Geometry: final body of the model. Coordinates: model frame, mm. Face numbers are marked on the shaded views. A direction names the side the tool comes from. Round coordinates to 2 decimals unless told otherwise and drop trailing zeros. Loops run counter-clockwise (first coordinate to the right, second up) from the corner with the lowest first, then second, coordinate; pieces in that order, holes last. Notation, with made-up numbers: (67, 89) -> (125, 89) arc R23 cw to (125, 112) -> close; hole circle Ø6 at (59.5, 40). An arc over 180 degrees is marked (long way). Answer in a Markdown table with one row per item.
```python
from build123d import *

# Parameters (mm, degrees)
BOSS_EXTRUDE1_DEPTH      = 1.5
BOSS_EXTRUDE2_DEPTH      = 6
BOSS_EXTRUDE2_DEPTH_BACK = 3
CUT_EXTRUDE1_DEPTH       = 13.69206445
CUT_EXTRUDE1_DEPTH_BACK  = 13.69206445


with BuildPart() as part:
    # Sketch1 → Boss-Extrude1 (new body)
    with BuildSketch(Plane(origin=(0, 0, 0), x_dir=(1, 0, 0), z_dir=(0, 1, 0))):
        Polygon((-0.635, 10.16), (0.635, 10.16), (1.27, 9.525), (1.27, 8.255), (0.635, 7.62), (1.27, 6.985), (1.27, 5.715), (0.635, 5.08), (1.27, 4.445), (1.27, 3.175), (0.635, 2.54), (1.27, 1.905), (1.27, 0.635), (0.635, 0), (1.27, -0.635), (1.27, -1.905), (0.635, -2.54), (1.27, -3.175), (1.27, -4.445), (0.635, -5.08), (-0.635, -5.08), (-1.27, -4.445), (-1.27, -3.175), (-0.635, -2.54), (-1.27, -1.905), (-1.27, -0.635), (-0.635, 0), (-1.27, 0.635), (-1.27, 1.905), (-0.635, 2.54), (-1.27, 3.175), (-1.27, 4.445), (-0.635, 5.08), (-1.27, 5.715), (-1.27, 6.985), (-0.635, 7.62), (-1.27, 8.255), (-1.27, 9.525), align=None)
    extrude(amount=BOSS_EXTRUDE1_DEPTH)

    # Sketch3 → Boss-Extrude2 (add, two sides: drawn at the far end of the back side and taken through both)
    with BuildSketch(Plane(origin=(0, 1.5, 0), x_dir=(1, 0, 0), z_dir=(0, 1, 0)).offset(-BOSS_EXTRUDE2_DEPTH_BACK)):
        Polygon((0.375, 9.39), (0.5, 9.265), (0.5, 8.515), (0.375, 8.39), (-0.375, 8.39), (-0.5, 8.515), (-0.5, 9.265), (-0.375, 9.39), align=None)
        Polygon((0.375, 6.85), (0.5, 6.725), (0.5, 5.975), (0.375, 5.85), (-0.375, 5.85), (-0.5, 5.975), (-0.5, 6.725), (-0.375, 6.85), align=None)
        Polygon((0.375, 4.31), (0.5, 4.185), (0.5, 3.435), (0.375, 3.31), (-0.375, 3.31), (-0.5, 3.435), (-0.5, 4.185), (-0.375, 4.31), align=None)
        Polygon((0.375, 1.77), (0.5, 1.645), (0.5, 0.895), (0.375, 0.77), (-0.375, 0.77), (-0.5, 0.895), (-0.5, 1.645), (-0.375, 1.77), align=None)
        Polygon((0.375, -0.77), (0.5, -0.895), (0.5, -1.645), (0.375, -1.77), (-0.375, -1.77), (-0.5, -1.645), (-0.5, -0.895), (-0.375, -0.77), align=None)
        Polygon((0.375, -3.31), (0.5, -3.435), (0.5, -4.185), (0.375, -4.31), (-0.375, -4.31), (-0.5, -4.185), (-0.5, -3.435), (-0.375, -3.31), align=None)
    extrude(amount=BOSS_EXTRUDE2_DEPTH + BOSS_EXTRUDE2_DEPTH_BACK)

    # Sketch4 → Cut-Extrude1 (cut, two sides: drawn at the far end of the back side and taken through both)
    with BuildSketch(Plane(origin=(0, 0, 0), x_dir=(1, 0, 0), z_dir=(0, 1, 0)).offset(-CUT_EXTRUDE1_DEPTH_BACK)):
        Polygon((0.635, 2.54), (-0.635, 2.54), (-3.551273802, 2.145414022), (-3.551273802, -5.54901255), (3.518391637, -6.305302341), (3.518391637, 1.323359901), align=None)
    extrude(amount=CUT_EXTRUDE1_DEPTH + CUT_EXTRUDE1_DEPTH_BACK, mode=Mode.SUBTRACT)


solid = part.part
```
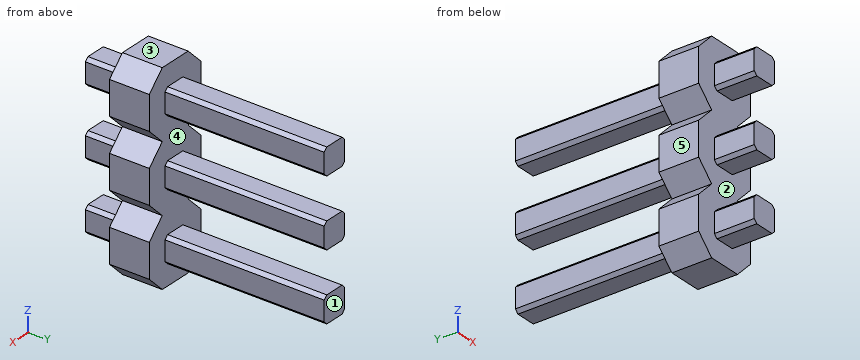
Item 1: Section query D-D, the plane z = -4. Output: boundary loops of the cut face in (x, y), and give its area (3 significant figures).
Ans:
| item | result |
|---|---|
| outline | (-1.27, 0) -> (-0.5, 0) -> (-0.5, -1.5) -> (0.5, -1.5) -> (0.5, 0) -> (1.27, 0) -> (1.27, 1.5) -> (0.5, 1.5) -> (0.5, 7.5) -> (-0.5, 7.5) -> (-0.5, 1.5) -> (-1.27, 1.5) -> close |
| area | 11.3 mm2 |
Item 2: Section query B-B, the plane x = 0.05. Output: boundary loops of the cut face in (y, z), and give its area (3 significant figures).
Ans:
| item | result |
|---|---|
| outline | (-1.5, -9.39) -> (0, -9.39) -> (0, -10.16) -> (1.5, -10.16) -> (1.5, -9.39) -> (7.5, -9.39) -> (7.5, -8.39) -> (1.5, -8.39) -> (1.5, -6.85) -> (7.5, -6.85) -> (7.5, -5.85) -> (1.5, -5.85) -> (1.5, -4.31) -> (7.5, -4.31) -> (7.5, -3.31) -> (1.5, -3.31) -> (1.5, -2.54) -> (0, -2.54) -> (0, -3.31) -> (-1.5, -3.31) -> (-1.5, -4.31) -> (0, -4.31) -> (0, -5.85) -> (-1.5, -5.85) -> (-1.5, -6.85) -> (0, -6.85) -> (0, -8.39) -> (-1.5, -8.39) -> close |
| area | 33.9 mm2 |
Item 3: Set-up query: the marked faces 1 and 2. Return all of +Z, -Z, +X, -X, +Y, -Y with unobstructed straight access to the full face (end or side cutting, diameter ignored); none if empty.
Ans:
| item | result |
|---|---|
| face 1 | +Z, -Z, +X, -X, +Y |
| face 2 | -Y |
Item 4: Section query A-A, the plane y = 5.5. Output: boundary loops of the cut face in (x, z) (3 decimals), and give its area (3 significant figures).
Ans:
| item | result |
|---|---|
| outline | (-0.5, -9.265) -> (-0.375, -9.39) -> (0.375, -9.39) -> (0.5, -9.265) -> (0.5, -8.515) -> (0.375, -8.39) -> (-0.375, -8.39) -> (-0.5, -8.515) -> close; (-0.5, -6.725) -> (-0.375, -6.85) -> (0.375, -6.85) -> (0.5, -6.725) -> (0.5, -5.975) -> (0.375, -5.85) -> (-0.375, -5.85) -> (-0.5, -5.975) -> close; (-0.5, -4.185) -> (-0.375, -4.31) -> (0.375, -4.31) -> (0.5, -4.185) -> (0.5, -3.435) -> (0.375, -3.31) -> (-0.375, -3.31) -> (-0.5, -3.435) -> close |
| area | 2.91 mm2 |
Item 5: First-contact query: P1, Ø0.8, axis at x = -0.5, z = -5, coming from the +Y side; P2, Ø0.6, axis at y = 4, z = -6.5, coming from the +X side; P3, Ø0.6, axis at y = -1, z = -6.5, coming from the -X side. Flat tips, straight axial feed; report the tip coordinate or a pass-through.
Ans:
| item | result |
|---|---|
| P1 | y = 1.5 |
| P2 | x = 0.5 |
| P3 | x = -0.5 |
Item 6: Section query C-C, the plane y = 1.25. Output: boundary loops of the cut face in (x, z) (3 decimals), and give its area (3 significant figures).
Ans:
| item | result |
|---|---|
| outline | (-1.27, -9.525) -> (-0.635, -10.16) -> (0.635, -10.16) -> (1.27, -9.525) -> (1.27, -8.255) -> (0.635, -7.62) -> (1.27, -6.985) -> (1.27, -5.715) -> (0.635, -5.08) -> (1.27, -4.445) -> (1.27, -3.175) -> (0.635, -2.54) -> (-0.635, -2.54) -> (-1.27, -3.175) -> (-1.27, -4.445) -> (-0.635, -5.08) -> (-1.27, -5.715) -> (-1.27, -6.985) -> (-0.635, -7.62) -> (-1.27, -8.255) -> close |
| area | 16.9 mm2 |
Item 7: Mould query, pull axis Z, two halves, no side actions, for the marked faces 3, 4 and 5. Classes: released by +Z, released by -Z, zero draft, split by the parting line, or undercut.
Ans:
| item | result |
|---|---|
| face 3 | released by +Z |
| face 4 | undercut |
| face 5 | zero draft |
Item 8: Ray query, L1, parallel to Z at x = 0.1, y = 3; L2, parallel to Z at x = 0.75, y = 0.5 (3 decimals); L3, parallel to Y at x = -0.4, z = -8.25. Return the intervals inside material, ascending.
Ans:
| item | result |
|---|---|
| L1 | -9.39 to -8.39, -6.85 to -5.85, -4.31 to -3.31 |
| L2 | -10.045 to -7.735, -7.505 to -5.195, -4.965 to -2.655 |
| L3 | 0 to 1.5 |
